Check sheet for the modelled part. Datum: model origin and axes. Units: mm. Face numbers are marked on the shaded views. A direction names the side the tool comes from. Give positions to 0.01 mm unless a question says otherwise; leave off trailing zeros. Write each loop counter-clockwise with the first axis right and the second up, starting at its lowest first coordinate (ties: lowest second). Pieces come first, ordered by that corner, then holes. Notation, with made-up numbers: M 77.5,58 L 109.5,58 A28 cw 109.5,96 Z; hole C -13,65 d5. An arc over 180 degrees is marked long. Write item = value, one per line. Start each with the question number.
1) Draft check along X on the marked faces 1, 2 and 3. Enter one of: pulls with the +X half, pulls with the -X half, needs draft (parallel to the pull), parting line crosses it, or undercut.
2) Sectioned sample at D-D, the plane y = 52. Record the cut outline in (x, z), then the cut area to 3 significant figures.
3) Sectioned sample at C-C, the plane z = 30. Count the separate pieces of the cut face and the enclosed holes in it, then the cut area to 3 significant figures.
4) Sectioned sample at B-B, the plane x = 30. Record the cut outline in (y, z), then the cut area to 3 significant figures.
5) Sectioned sample at A-A, the plane y = 71.5. Record the cut outline in (x, z), then the cut area to 3 significant figures.
6) Scan lines: L1, parallel to Y at x = 0, z = 30; L2, parallel to Z at x = 0.15, y = 12; L3, parallel to Y at x = 11, z = 30. Record each from-to range of solid material in increasing order.
7) Gauge pin test, flat ends, axial feed: pin 1 (9.5 mm diameter, centred on y = 12, z = 30, fed in from -X); pin 2 (1 mm diameter, centred on x = -1, y = 58.5, fed in from -Z); pin 3 (3 mm diameter, centred on y = 59, z = 13.5, fed in from +X); pin 4 (19 mm diameter, centred on x = 30, z = 30, fed in from -Y). Record the tip position at first contact, or that the pin passes through.
8) Set-up check for the marked faces 4, 5 and 6: record each of +Z, -Z, +X, -X, +Y, -Y from which the full face is reachable in a straight line by a thin tool's end or side.
from build123d import *

# Parameters (mm, degrees)
BOSS_EXTRUDE1_DEPTH     = 60
CUT_EXTRUDE1_DEPTH      = 121.453310457
CUT_EXTRUDE1_DEPTH_BACK = 121.453310457
SKETCH2_R               = 6
SKETCH3_R               = 17.6
CUT_EXTRUDE2_DEPTH      = 78
CUT_EXTRUDE4_REACH      = 122.453
CUT_EXTRUDE4_END_RADIUS = 17.6
SKETCH5_R               = 4.1
CUT_EXTRUDE6_START      = 53
SKETCH6_R               = 8
CUT_EXTRUDE6_DEPTH      = 50
SKETCH7_W               = 12
SKETCH7_H               = 90
BOSS_EXTRUDE4_DEPTH     = 3
CUT_EXTRUDE7_DEPTH      = 121.453310457
CUT_EXTRUDE7_DEPTH_BACK = 121.453310457
SKETCH5_2_R             = 4.1
CHAMFER1_SIZE           = 1


with BuildPart() as part:
    # Sketch1 → Boss-Extrude1 (new body)
    with BuildSketch(Plane.XY):
        Polygon((0, 0), (0, 90), (53, 90), (53, 67), (5, 0), align=None)
    extrude(amount=BOSS_EXTRUDE1_DEPTH)

    # Sketch2 → Cut-Extrude1 (cut, two sides: drawn at the far end of the back side and taken through both)
    with BuildSketch(Plane(origin=(0, 0, 0), x_dir=(1, 0, 0), z_dir=(0, 1, 0)).offset(-CUT_EXTRUDE1_DEPTH_BACK)):
        with Locations(Location((30, -30, 0), (0, 0, 180))):
            Circle(SKETCH2_R)
    extrude(amount=CUT_EXTRUDE1_DEPTH + CUT_EXTRUDE1_DEPTH_BACK, mode=Mode.SUBTRACT)

    # Sketch3 → Cut-Extrude2 (cut)
    with BuildSketch(Plane(origin=(0, 0, 0), x_dir=(1, 0, 0), z_dir=(0, 1, 0))):
        with Locations(Location((30, -30, 0), (0, 0, 180))):
            Circle(SKETCH3_R)
    extrude(amount=CUT_EXTRUDE2_DEPTH, mode=Mode.SUBTRACT)

    # Cut-Extrude4: up to this cylinder (the profile starts outside it)
    cut_extrude4_end = Plane(origin=(30, 32, 30), z_dir=(0, -1, 0)) * Cylinder(CUT_EXTRUDE4_END_RADIUS, 321.106, mode=Mode.PRIVATE)
    # Sketch5 → Cut-Extrude4 (cut, up to the surface)
    with BuildSketch(Plane(origin=(0, 0, 0), x_dir=(0, 0, -1), z_dir=(1, 0, 0)), mode=Mode.PRIVATE) as cut_extrude4_sk1:
        with Locations(Location((-30, 12, 0), (0, 0, 194.678469959))):
            Circle(SKETCH5_R)
    cut_extrude4_tool1 = extrude(cut_extrude4_sk1.sketch, amount=CUT_EXTRUDE4_REACH, mode=Mode.PRIVATE) - cut_extrude4_end
    add(cut_extrude4_tool1.solids().sort_by_distance((0, 12, 30))[0], mode=Mode.SUBTRACT)
    # Sketch5 → Cut-Extrude4 (cut, up to the surface)
    with BuildSketch(Plane(origin=(0, 0, 0), x_dir=(0, 0, -1), z_dir=(1, 0, 0)), mode=Mode.PRIVATE) as cut_extrude4_sk2:
        with Locations(Location((-30, 52, 0), (0, 0, 180))):
            Circle(SKETCH5_R)
    cut_extrude4_tool2 = extrude(cut_extrude4_sk2.sketch, amount=CUT_EXTRUDE4_REACH, mode=Mode.PRIVATE) - cut_extrude4_end
    add(cut_extrude4_tool2.solids().sort_by_distance((0, 52, 30))[0], mode=Mode.SUBTRACT)

    # Sketch6 → Cut-Extrude6 (cut)
    with BuildSketch(Plane(origin=(0, 0, 0), x_dir=(0, 0, -1), z_dir=(1, 0, 0)).offset(CUT_EXTRUDE6_START)):
        with Locations((-30, 52)):
            Circle(SKETCH6_R)
        with Locations(Location((-30, 12, 0), (0, 0, 6.976713047))):
            Circle(SKETCH6_R)
    extrude(amount=-CUT_EXTRUDE6_DEPTH, mode=Mode.SUBTRACT)

    # Sketch7 → Boss-Extrude4 (add)
    with BuildSketch(Plane(origin=(0, 0, 0), x_dir=(0, 0, -1), z_dir=(1, 0, 0))):
        with Locations((-30, 45)):
            Rectangle(SKETCH7_W, SKETCH7_H)
    extrude(amount=-BOSS_EXTRUDE4_DEPTH)

    # Sketch5<2> → Cut-Extrude7 (cut, two sides: drawn at the far end of the back side and taken through both)
    with BuildSketch(Plane(origin=(0, 0, 0), x_dir=(0, 0, -1), z_dir=(1, 0, 0)).offset(-CUT_EXTRUDE7_DEPTH_BACK)):
        with Locations(Location((-30, 12, 0), (0, 0, 180))):
            Circle(SKETCH5_2_R)
        with Locations(Location((-30, 52, 0), (0, 0, 180))):
            Circle(SKETCH5_2_R)
    extrude(amount=CUT_EXTRUDE7_DEPTH + CUT_EXTRUDE7_DEPTH_BACK, mode=Mode.SUBTRACT)

    # Chamfer1
    chamfer1_edges = [part.edges().sort_by_distance(p)[0] for p in [
        (-3, 45, 36),
        (-3, 45, 24),
    ]]
    chamfer(chamfer1_edges, length=CHAMFER1_SIZE)


solid = part.part
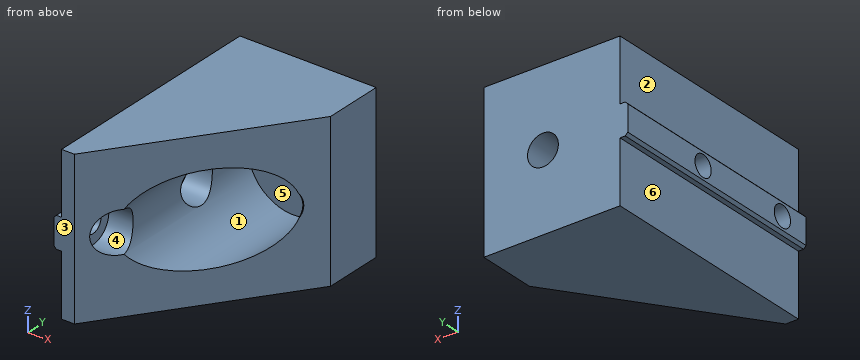
Data:
q1.face_1 = undercut
q1.face_2 = pulls with the -X half
q1.face_3 = needs draft
q2.outline = M -3,25 L -2,24 L 0,24 L 0,0 L 42.25,0 L 42.25,17.37 A17.6 cw 14.32,22 L 3,22 L 3,25.9 L -3,25.9 Z; M -3,34.1 L 3,34.1 L 3,38 L 14.32,38 A17.6 cw 42.25,42.63 L 42.25,60 L 0,60 L 0,36 L -2,36 L -3,35 Z
q2.area = 1,480 mm2
q3.separate_pieces = 4
q3.enclosed_holes = 0
q3.area = 1,390 mm2
q4.outline = M 34.9,0 L 90,0 L 90,24 L 78,24 L 78,12.4 L 34.9,12.4 Z; M 34.9,47.6 L 78,47.6 L 78,36 L 90,36 L 90,60 L 34.9,60 Z
q4.area = 1,640 mm2
q5.outline = M -3,25 L -2,24 L 0,24 L 0,0 L 53,0 L 53,60 L 0,60 L 0,36 L -2,36 L -3,35 Z; hole C 30,30 d35.2
q5.area = 2,240 mm2
q6.L1 = 0 to 7.9, 16.1 to 47.9, 56.1 to 90
q6.L2 = 0 to 25.9, 34.1 to 60
q6.L3 = 20 to 44, 60 to 90
q7.pin_1 = -3
q7.pin_2 = 24
q7.pin_3 = 48.34
q7.pin_4 = 78
q8.face_4 = +X
q8.face_5 = -Y
q8.face_6 = -Z, -X, +Y, -Y
